from build123d import *

# Parameters (mm, degrees)
SKETCH1_W            = 68.58
SKETCH1_H            = 88.9
BOSS_EXTRUDE1_DEPTH  = 96.52
SKETCH2_W            = 58.42
SKETCH2_H            = 81.28
CUT_EXTRUDE1_DEPTH   = 149.062611081
SKETCH3_W            = 20.32
SKETCH3_H            = 12.7
BOSS_EXTRUDE2_DEPTH  = 38.1
SKETCH4_W            = 20.32
SKETCH4_H            = 19.05
BOSS_EXTRUDE3_DEPTH  = 12.7
SKETCH5_W            = 20.32
SKETCH5_H            = 9.525
BOSS_EXTRUDE4_DEPTH  = 7.62
CUT_EXTRUDE2_DEPTH   = 141.804001364
SKETCH7_W            = 68.58
SKETCH7_H            = 5.08
BOSS_EXTRUDE5_DEPTH  = 7.62
SKETCH8_W            = 68.58
SKETCH8_H            = 3.556
BOSS_EXTRUDE6_DEPTH  = 7.62
SKETCH9_W            = 68.58
SKETCH9_H            = 3.556
BOSS_EXTRUDE7_DEPTH  = 7.62
SKETCH10_W           = 40.64
SKETCH10_H           = 12.7
BOSS_EXTRUDE8_DEPTH  = 35.56
SKETCH11_R           = 5.715
CUT_EXTRUDE3_DEPTH   = 140.7147774
BOSS_EXTRUDE9_START  = 2.032
SKETCH13_W           = 40.64
SKETCH13_H           = 35.56
SKETCH13_R           = 5.715
BOSS_EXTRUDE9_DEPTH  = 2.032
SKETCH15_W           = 20.32
SKETCH15_H           = 12.7
BOSS_EXTRUDE10_DEPTH = 7.62
BOSS_EXTRUDE11_START = 12.7
SKETCH16_R           = 5.715
BOSS_EXTRUDE11_DEPTH = 12.7


with BuildPart() as part:
    # Sketch1 → Boss-Extrude1 (new body)
    with BuildSketch(Plane(origin=(0, 0, 0), x_dir=(-1, 0, 0), z_dir=(0, 1, 0))):
        with Locations((34.29, 44.45)):
            Rectangle(SKETCH1_W, SKETCH1_H)
    extrude(amount=BOSS_EXTRUDE1_DEPTH)

    # Sketch2 → Cut-Extrude1 (cut, through all)
    with BuildSketch(Plane.XY.offset(88.9)):
        with Locations((-34.29, 48.26)):
            Rectangle(SKETCH2_W, SKETCH2_H)
    extrude(amount=-CUT_EXTRUDE1_DEPTH, mode=Mode.SUBTRACT)

    # Sketch3 → Boss-Extrude2 (add)
    with BuildSketch(Plane(origin=(0, 7.62, 0), x_dir=(-1, 0, 0), z_dir=(0, 1, 0))):
        with Locations((34.29, 69.85)):
            Rectangle(SKETCH3_W, SKETCH3_H)
    extrude(amount=BOSS_EXTRUDE2_DEPTH)

    # Sketch4 → Boss-Extrude3 (add)
    with BuildSketch(Plane(origin=(0, 0, 63.5), x_dir=(1, 0, 0), z_dir=(0, 0, -1))):
        with Locations((-34.29, -17.145)):
            Rectangle(SKETCH4_W, SKETCH4_H)
    extrude(amount=BOSS_EXTRUDE3_DEPTH)

    # Sketch5 → Boss-Extrude4 (add)
    with BuildSketch(Plane(origin=(0, 0, 50.8), x_dir=(1, 0, 0), z_dir=(0, 0, -1))):
        with Locations((-34.29, -12.3825)):
            Rectangle(SKETCH5_W, SKETCH5_H)
    extrude(amount=BOSS_EXTRUDE4_DEPTH)

    # Sketch6 → Cut-Extrude2 (cut, through all)
    with BuildSketch(Plane.XY.offset(76.2)):
        with BuildLine():
            Line((-37.973, 42.164), (-30.607, 42.164))
            ThreePointArc((-30.607, 42.164), (-28.117747737, 37.211), (-30.607, 32.258))
            Line((-30.607, 32.258), (-37.973, 32.258))
            ThreePointArc((-37.973, 32.258), (-40.462252263, 37.211), (-37.973, 42.164))
        make_face()
    extrude(amount=-CUT_EXTRUDE2_DEPTH, mode=Mode.SUBTRACT)

    # Sketch7 → Boss-Extrude5 (add)
    with BuildSketch(Plane.XZ):
        with Locations((-34.29, 74.676)):
            Rectangle(SKETCH7_W, SKETCH7_H)
        with Locations((-34.29, 36.576)):
            Rectangle(SKETCH7_W, SKETCH7_H)
    extrude(amount=BOSS_EXTRUDE5_DEPTH)

    # Sketch8 → Boss-Extrude6 (add)
    with BuildSketch(Plane(origin=(0, 0, 72.136), x_dir=(1, 0, 0), z_dir=(0, 0, -1))):
        with Locations((-34.29, 5.842)):
            Rectangle(SKETCH8_W, SKETCH8_H)
    extrude(amount=BOSS_EXTRUDE6_DEPTH)

    # Sketch9 → Boss-Extrude7 (add)
    with BuildSketch(Plane(origin=(0, 0, 34.036), x_dir=(1, 0, 0), z_dir=(0, 0, -1))):
        with Locations((-34.29, 5.842)):
            Rectangle(SKETCH9_W, SKETCH9_H)
    extrude(amount=BOSS_EXTRUDE7_DEPTH)

    # Sketch10 → Boss-Extrude8 (add)
    with BuildSketch(Plane.XZ.offset(-88.9)):
        with Locations((-34.29, 67.818)):
            Rectangle(SKETCH10_W, SKETCH10_H)
    extrude(amount=BOSS_EXTRUDE8_DEPTH)

    # Sketch11 → Cut-Extrude3 (cut, through all)
    with BuildSketch(Plane.XY.offset(74.168)):
        with Locations((-34.29, 66.04)):
            Circle(SKETCH11_R)
    extrude(amount=-CUT_EXTRUDE3_DEPTH, mode=Mode.SUBTRACT)

    # Sketch13 → Boss-Extrude9 (add)
    with BuildSketch(Plane.XY.offset(74.168).offset(BOSS_EXTRUDE9_START)):
        with Locations((-34.29, 71.12)):
            Rectangle(SKETCH13_W, SKETCH13_H)
        with Locations((-34.29, 66.04)):
            Circle(SKETCH13_R, mode=Mode.SUBTRACT)
    extrude(amount=-BOSS_EXTRUDE9_DEPTH)

    # Sketch15 → Boss-Extrude10 (add)
    with BuildSketch(Plane(origin=(0, 45.72, 0), x_dir=(-1, 0, 0), z_dir=(0, 1, 0))):
        with Locations((34.29, 69.85)):
            Rectangle(SKETCH15_W, SKETCH15_H)
    extrude(amount=BOSS_EXTRUDE10_DEPTH)

    # Sketch16 → Boss-Extrude11 (add)
    with BuildSketch(Plane.XY.offset(76.2).offset(BOSS_EXTRUDE11_START)):
        Polygon((-54.61, 88.9), (-13.97, 88.9), (-13.97, 53.34), (-24.13, 53.34), (-24.13, 7.62), (-44.45, 7.62), (-44.45, 53.34), (-54.61, 53.34), align=None)
        with Locations((-34.29, 66.04)):
            Circle(SKETCH16_R, mode=Mode.SUBTRACT)
        with BuildLine():
            Line((-37.973, 42.164), (-30.607, 42.164))
            ThreePointArc((-30.607, 42.164), (-28.117747737, 37.211), (-30.607, 32.258))
            Line((-30.607, 32.258), (-37.973, 32.258))
            ThreePointArc((-37.973, 32.258), (-40.462252263, 37.211), (-37.973, 42.164))
        make_face(mode=Mode.SUBTRACT)
    extrude(amount=-BOSS_EXTRUDE11_DEPTH)


solid = part.part
Check sheet for the modelled part. Datum: model origin and axes. Units: mm. A direction names the side the tool comes from. Coordinates: 2 decimals unless noted, no trailing zeros. Loops run counter-clockwise (first coordinate to the right, second up) from the corner with the lowest first, then second, coordinate; pieces in that order, holes last. Notation, with made-up numbers: (-21, -29) -> (28, -29) arc R13 ccw to (28, -15) -> close; hole circle Ø4 at (87.5, 13). An arc over 180 degrees is marked (long way). Write item = value, one per line. Start each with the question number.
1. Draft check along Y on faces 1 (the flat face through (-34, 0, 83)), 2 (the flat face through (-63.5, 48, 45)), 3 (the flat face through (-35, -4, 39.116)). Enter one of: released by +Y, released by -Y, zero draft, split by the parting line, or undercut.
2. Section check B-B on z = 69.5. Give the number of separate pieces and of enclosed holes in the cut face, then the cut area to 3 significant figures.
3. Section check A-A on z = 29.5. Record the cut outline in (x, y).
4. Depth check by flat-ended pin: P1, Ø7.5, axis at x = -30.5, y = 12, coming from the -Z side; P2, Ø10, axis at x = -27.5, z = 52.5, coming from the -Y side; P3, Ø4.5, axis at x = -35, y = -2.5, coming from the -Z side. Enter the tip coordinate at first touch or a pass-through.
5. Material ranges on line 1 (X direction, y = 54, z = 67); line 2 (X direction, y = 66, z = 82); line 3 (X direction, y = 44, z = 74), recorded low to high.
6. Section check C-C on x = -57. Record the cut outline in (y, z).
7. Section check D-D on y = 66.04. Record the cut outline in (x, z) (3 decimals), then the cut area to 3 significant figures.
8. Tool access check on faces 4 (the flat face through (-34, 32.258, 76)), 5 (the flat face through (-35, -4.064, 30)), 6 (the flat face through (0, 45, 45)), 7 (the flat face through (-34, 12, 43.18)), 8 (the flat face through (-35, -6, 26.416)). Record the directions out of +Z, -Z, +X, -X, +Y, -Y that give a thin tool (end or side, any length) a straight path to the whole face; none if there is none.
Responses:
q1.face_1 = released by -Y
q1.face_2 = undercut
q1.face_3 = zero draft
q2.separate_pieces = 2
q2.enclosed_holes = 4
q2.area = 4,280 mm2
q3.outline = (-68.58, -7.62) -> (0, -7.62) -> (0, -4.06) -> (-68.58, -4.06) -> close; (-68.58, 0) -> (0, 0) -> (0, 96.52) -> (-68.58, 96.52) -> close; hole (-63.5, 7.62) -> (-5.08, 7.62) -> (-5.08, 88.9) -> (-63.5, 88.9) -> close
q4.P1 = 43.18
q4.P2 = 0
q4.P3 = 26.42
q5.line_1 = -68.58 to -63.5, -54.61 to -13.97, -5.08 to 0
q5.line_2 = -68.58 to -63.5, -54.61 to -40, -28.58 to -13.97, -5.08 to 0
q5.line_3 = -68.58 to -63.5, -44.45 to -24.13, -5.08 to 0
q6.outline = (-7.62, 26.42) -> (-4.06, 26.42) -> (-4.06, 34.04) -> (0, 34.04) -> (0, 0) -> (7.62, 0) -> (7.62, 88.9) -> (0, 88.9) -> (0, 77.22) -> (-7.62, 77.22) -> (-7.62, 64.52) -> (-4.06, 64.52) -> (-4.06, 72.14) -> (0, 72.14) -> (0, 39.12) -> (-7.62, 39.12) -> close; (88.9, 0) -> (96.52, 0) -> (96.52, 88.9) -> (88.9, 88.9) -> close
q7.outline = (-68.58, 0) -> (-63.5, 0) -> (-63.5, 88.9) -> (-68.58, 88.9) -> close; (-54.61, 61.468) -> (-40.005, 61.468) -> (-40.005, 88.9) -> (-54.61, 88.9) -> close; (-28.575, 61.468) -> (-13.97, 61.468) -> (-13.97, 88.9) -> (-28.575, 88.9) -> close; (-5.08, 0) -> (0, 0) -> (0, 88.9) -> (-5.08, 88.9) -> close
q7.area = 1,700 mm2
q8.face_4 = +Z, -Z
q8.face_5 = -Z, +X, -X
q8.face_6 = +Z, -Z, +X, +Y, -Y
q8.face_7 = -Z
q8.face_8 = -Z, +X, -X, -Y
